from build123d import *

# Parameters (mm, degrees)
EXTRUDE_1_DEPTH     = 480
SKETCH_2_R          = 1.5
SKETCH_2_R_2        = 2
CUT_EXTRUDE_1_DEPTH = 481.59364332
CHAMFER_1_SIZE      = 1


with BuildPart() as part:
    # ｽｹｯﾁ1 → ﾎﾞｽ - 押し出し1 (new body)
    with BuildSketch(Plane.XY):
        Polygon((0, 8), (-2.5, 8), (-2.5, -2), (22.5, -2), (22.5, 8), (20, 8), (20, 0), (0, 0), align=None)
    extrude(amount=EXTRUDE_1_DEPTH)

    # ｽｹｯﾁ2 → ｶｯﾄ - 押し出し1 (cut, through all)
    with BuildSketch(Plane(origin=(0, 0, 0), x_dir=(1, 0, 0), z_dir=(0, 1, 0))):
        with Locations(Location((10, -477, 0), (0, 0, 270))):
            Circle(SKETCH_2_R)
        with Locations(Location((10, -440, 0), (0, 0, 270))):
            Circle(SKETCH_2_R_2)
        with Locations(Location((10, -360, 0), (0, 0, 270))):
            Circle(SKETCH_2_R_2)
        with Locations(Location((10, -280, 0), (0, 0, 270))):
            Circle(SKETCH_2_R_2)
        with Locations(Location((10, -200, 0), (0, 0, 270))):
            Circle(SKETCH_2_R_2)
        with Locations(Location((10, -120, 0), (0, 0, 270))):
            Circle(SKETCH_2_R_2)
        with Locations(Location((10, -40, 0), (0, 0, 270))):
            Circle(SKETCH_2_R_2)
        with Locations(Location((10, -3, 0), (0, 0, 270))):
            Circle(SKETCH_2_R)
    extrude(amount=-CUT_EXTRUDE_1_DEPTH, mode=Mode.SUBTRACT)

    # 面取り1
    chamfer_1_edges = [part.edges().sort_by_distance(p)[0] for p in [
        (10, 0, 438),
        (10, 0, 358),
        (10, 0, 278),
        (10, 0, 198),
        (10, 0, 118),
        (10, 0, 38),
    ]]
    chamfer(chamfer_1_edges, length=CHAMFER_1_SIZE)


solid = part.part
Could you check a few things on this model? Use its own coordinates, in mm. A direction names the side the tool comes from. Give positions to 0.01 mm unless a question says otherwise; leave off trailing zeros. Order: outer loops, then holes, each group sorted by start corner. A loop starts at its lowest first (then second) coordinate and runs counter-clockwise, first axis right, second up. Notation, with made-up numbers: (-33, -32) - (-11, -32) arc R33 ccw to (-11, 5) - close; hole circle Ø9 at (24.5, 73.5). An arc over 180 degrees is marked (long way). Return JSON: item names as keys, results as strings. Group by question number.
Q1. Which directions (+Z, -Z, +X, -X, +Y, -Y) give clear straight access to the entire face, cutting with the end or side of a thin tool? Please do faces 1 (the face through (9.8, -0.3, 0)), 2 (the face through (0, 4, 237)).
Q2. Will this pin go through, and if not, where does the flat tip stop? pin 1 Ø6.5 at (x, z) = (10, 40) entering from +Y.
Q3. Suppose I cut it at B-B, the plane z = 137. Please give me the cut outline in (x, y).
Q4. Suppose I cut it at A-A, the plane y = 3. Please give me the cut outline in (x, z).
Q5. Thinking about a two-plate mould opening in X: for faces 3 (the face through (10, 0, 237)), 4 (the face through (22.5, 3, 237)), 5 (the face through (9.8, -0.3, 480)), 6 (the face through (-2.5, 3, 237)), which applies, pulls with the +X half, pulls with the -X half, needs draft (parallel to the pull), parting line crosses it, or undercut?
Q6. Please list where these lines run through material, in increasing order: line 1 along X through (y, z) = (-1.35, 440); line 2 along X through (y, z) = (1.5, 99); line 3 along Y through (x, z) = (12.5, 351.5). Write a range as [from, to].
Resolved:
{
 "1": {"face 1": "-Z, +X, -X, +Y, -Y", "face 2": "+Z, -Z, +Y"},
 "2": {"pin 1": "stops at y = 0"},
 "3": {"outline": "(-2.5, -2) - (22.5, -2) - (22.5, 8) - (20, 8) - (20, 0) - (0, 0) - (0, 8) - (-2.5, 8) - close"},
 "4": {"outline": "(-2.5, 0) - (0, 0) - (0, 480) - (-2.5, 480) - close; (20, 0) - (22.5, 0) - (22.5, 480) - (20, 480) - close"},
 "5": {"face 3": "undercut", "face 4": "pulls with the +X half", "face 5": "needs draft", "face 6": "pulls with the -X half"},
 "6": {"line 1": "x = [-2.5, 8], [12, 22.5]", "line 2": "x = [-2.5, 0], [20, 22.5]", "line 3": "y = [-2, 0]"}
}
